Geometry: final body of the model. Coordinates: model frame, mm. A direction names the side the tool comes from. Give positions to 0.01 mm unless a question says otherwise; leave off trailing zeros. Loops run counter-clockwise (first coordinate to the right, second up) from the corner with the lowest first, then second, coordinate; pieces in that order, holes last. Notation, with made-up numbers: (38.25, 3) - (56.25, 3) arc R28 cw to (56.25, 29) - close; hole circle Ø7 at (69, 27). An arc over 180 degrees is marked (long way). Answer in a Markdown table with one row per item.
from build123d import *

# Parameters (mm, degrees)
ESQUISSE1_W             = 7
ESQUISSE1_H             = 113
ESQUISSE1_W_2           = 120
ESQUISSE1_H_2           = 7
BOSS_EXTRU_2_DEPTH      = 40
ESQUISSE4_W             = 113
ESQUISSE4_H             = 10
BOSS_EXTRU_8_DEPTH      = 115
ENL_V_MAT_EXTRU_2_DEPTH = 115
ESQUISSE2_R             = 1
ENL_V_MAT_EXTRU_4_DEPTH = 115
ESQUISSE7_R             = 1
ENL_V_MAT_EXTRU_5_DEPTH = 115
ESQUISSE8_R             = 1
ENL_V_MAT_EXTRU_6_DEPTH = 115
ESQUISSE9_R             = 1
ENL_V_MAT_EXTRU_7_DEPTH = 115
ESQUISSE10_R            = 1
ENL_V_MAT_EXTRU_8_DEPTH = 20


with BuildPart() as part:
    # Esquisse1 → Boss.-Extru.2 (new body)
    with BuildSketch(Plane.XY):
        with Locations((23.75751598, 59.836675468)):
            Rectangle(ESQUISSE1_W, ESQUISSE1_H)
        with Locations((-32.74248402, -0.163324532)):
            Rectangle(ESQUISSE1_W_2, ESQUISSE1_H_2)
    extrude(amount=BOSS_EXTRU_2_DEPTH)

    # Esquisse4 → Boss.-Extru.8 (add)
    with BuildSketch(Plane(origin=(0, 3.336675468, 0), x_dir=(1, 0, 0), z_dir=(0, 1, 0))):
        with Locations((-36.24248402, -35)):
            Rectangle(ESQUISSE4_W, ESQUISSE4_H)
    extrude(amount=BOSS_EXTRU_8_DEPTH)

    # Esquisse6 → Enlèv. mat.-Extru.2 (cut)
    with BuildSketch(Plane.XY.offset(40)):
        Polygon((20.25751598, 116.336675468), (-92.74248402, 3.336675468), (-92.74248402, 118.336675468), (20.25751598, 118.336675468), align=None)
    extrude(amount=-ENL_V_MAT_EXTRU_2_DEPTH, mode=Mode.SUBTRACT)

    # Esquisse2 → Enlèv. mat.-Extru.4 (cut)
    with BuildSketch(Plane(origin=(0, 3.336675468, 0), x_dir=(1, 0, 0), z_dir=(0, 1, 0))):
        with Locations(Location((-57.74248402, -15, 0), (0, 0, 180))):  # turned: the seam where the file's is
            Circle(ESQUISSE2_R)
    extrude(amount=-ENL_V_MAT_EXTRU_4_DEPTH, mode=Mode.SUBTRACT)

    # Esquisse7 → Enlèv. mat.-Extru.5 (cut)
    with BuildSketch(Plane(origin=(0, 3.336675468, 0), x_dir=(1, 0, 0), z_dir=(0, 1, 0))):
        with Locations(Location((-9.74248402, -15, 0), (0, 0, 180))):  # turned: the seam where the file's is
            Circle(ESQUISSE7_R)
    extrude(amount=-ENL_V_MAT_EXTRU_5_DEPTH, mode=Mode.SUBTRACT)

    # Esquisse8 → Enlèv. mat.-Extru.6 (cut)
    with BuildSketch(Plane.ZY.offset(-20.25751598)):
        with Locations((15, 81.336675468)):
            Circle(ESQUISSE8_R)
    extrude(amount=-ENL_V_MAT_EXTRU_6_DEPTH, mode=Mode.SUBTRACT)

    # Esquisse9 → Enlèv. mat.-Extru.7 (cut)
    with BuildSketch(Plane.ZY.offset(-20.25751598)):
        with Locations((15, 33.336675468)):
            Circle(ESQUISSE9_R)
    extrude(amount=-ENL_V_MAT_EXTRU_7_DEPTH, mode=Mode.SUBTRACT)

    # Esquisse10 → Enlèv. mat.-Extru.8 (cut)
    with BuildSketch(Plane(origin=(0, 0, 30), x_dir=(-1, 0, 0), z_dir=(0, 0, -1))):
        with Locations((14.74248402, 38.336675468)):
            Circle(ESQUISSE10_R)
    extrude(amount=-ENL_V_MAT_EXTRU_8_DEPTH, mode=Mode.SUBTRACT)


solid = part.part
Q1. First-contact query: pin 1 (12 mm diameter, centred on x = -51.5, z = 22.5, fed in from +Y); pin 2 (15 mm diameter, centred on y = 62.5, z = 22, fed in from -X); pin 3 (1.5 mm diameter, centred on x = -51, y = 23, fed in from -Z); pin 4 (1.8 mm diameter, centred on x = -57.74, z = 15, fed in from -Y). Flat tips, straight axial feed; report the tip coordinate or a pass-through.
Check values:
| item | result |
|---|---|
| pin 1 | y = 3.34 |
| pin 2 | x = 20.26 |
| pin 3 | z = 30 |
| pin 4 | through |
Q2. Cut plane B-B (y = 73). Output: boundary loops of the cut face in (x, z).
Check values:
| item | result |
|---|---|
| outline | (-23.08, 30) - (20.26, 30) - (20.26, 0) - (27.26, 0) - (27.26, 40) - (-23.08, 40) - close |
Q3. Cut plane A-A (z = 28.5). Output: boundary loops of the cut face in (x, y), and give its area (3 significant figures).
Check values:
| item | result |
|---|---|
| outline | (-92.74, -3.66) - (27.26, -3.66) - (27.26, 116.34) - (20.26, 116.34) - (20.26, 3.34) - (-92.74, 3.34) - close |
| area | 1,630 mm² |
Q4. Material intervals for line 1 along Y through (x, z) = (24, 15); line 2 along X through (y, z) = (24.5, 6); line 3 along Y through (x, z) = (-67, 26.5), sorted ascending.
Check values:
| item | result |
|---|---|
| line 1 | -3.66 to 32.34, 34.34 to 80.34, 82.34 to 116.34 |
| line 2 | 20.26 to 27.26 |
| line 3 | -3.66 to 3.34 |
Q5. Reachability of faces 1 (the flat face through (-35.45, 60.63, 35.07)), 2 (the flat face through (-12, 34, 30)) from +Z, -Z, +X, -X, +Y, -Y: full face, straight path, thin tool, end or side. Return the list, or none.
Check values:
| item | result |
|---|---|
| face 1 | +Z, -Z, -X, +Y |
| face 2 | -Z, -X, +Y |
